Can you work these out from the drawing? Everything is in mm from the part's minimum corner. Round coordinates to 2 decimals unless told otherwise and drop trailing zeros. Write each loop counter-clockwise with the first axis right and the second up, starting at its lowest first coordinate (ties: lowest second). Pieces come first, ordered by that corner, then holes.
Q1. If we section it at C-C (x = 48.5): Please give me the cut outline in (y, z), plus the area to 3 significant figures.
Q2. If we section it at D-D (x = 9): Please give me the cut outline in (y, z).
Q3. I'm going to push flat-ended pins straight in: pin 1 Ø8 at (x, y) = (28, 16) entering from +Z; pin 2 Ø1.2 at (y, z) = (19.5, 20) entering from +X; pin 3 Ø2.5 at (x, y) = (57, 21.5) entering from +Z. Where does each tip first touch, or does it pass through?
Q4. Please list where these lines run through material, in increasing order: line 1 along Y through (x, z) = (65.2, 20.3); line 2 along Y through (x, z) = (8, 16); line 3 along X through (y, z) = (19.75, 20.5).
Q5. If we section it at B-B (y = 19.5): Please give me the cut outline in (x, z).
Q6. If we section it at A-A (z = 20.3): Please give me the cut outline in (x, y), plus the area to 3 significant figures.
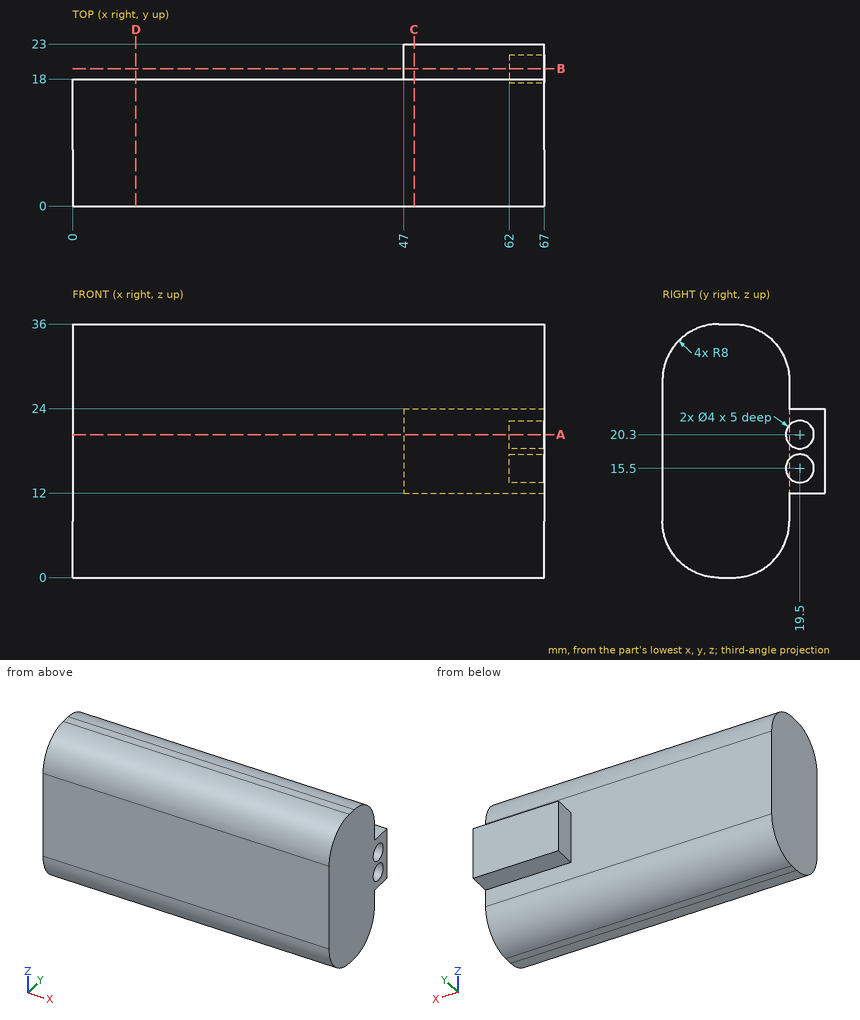
A:
1. outline: (0, 8) arc R8 ccw to (8, 0) - (10, 0) arc R8 ccw to (18, 8) - (18, 12) - (23, 12) - (23, 24) - (18, 24) - (18, 28) arc R8 ccw to (10, 36) - (8, 36) arc R8 ccw to (0, 28) - close
1. area: 653 mm2
2. outline: (0, 8) arc R8 ccw to (8, 0) - (10, 0) arc R8 ccw to (18, 8) - (18, 28) arc R8 ccw to (10, 36) - (8, 36) arc R8 ccw to (0, 28) - close
3. pin 1: stops at z = 35.75
3. pin 2: stops at x = 62
3. pin 3: stops at z = 24
4. line 1: y = 0 to 17.5, 21.5 to 23
4. line 2: y = 0 to 18
4. line 3: x = 47 to 62
5. outline: (47, 12) - (67, 12) - (67, 13.5) - (62, 13.5) - (62, 17.5) - (67, 17.5) - (67, 18.3) - (62, 18.3) - (62, 22.3) - (67, 22.3) - (67, 24) - (47, 24) - close
6. outline: (0, 0) - (67, 0) - (67, 17.5) - (62, 17.5) - (62, 21.5) - (67, 21.5) - (67, 23) - (47, 23) - (47, 18) - (0, 18) - close
6. area: 1,290 mm2
